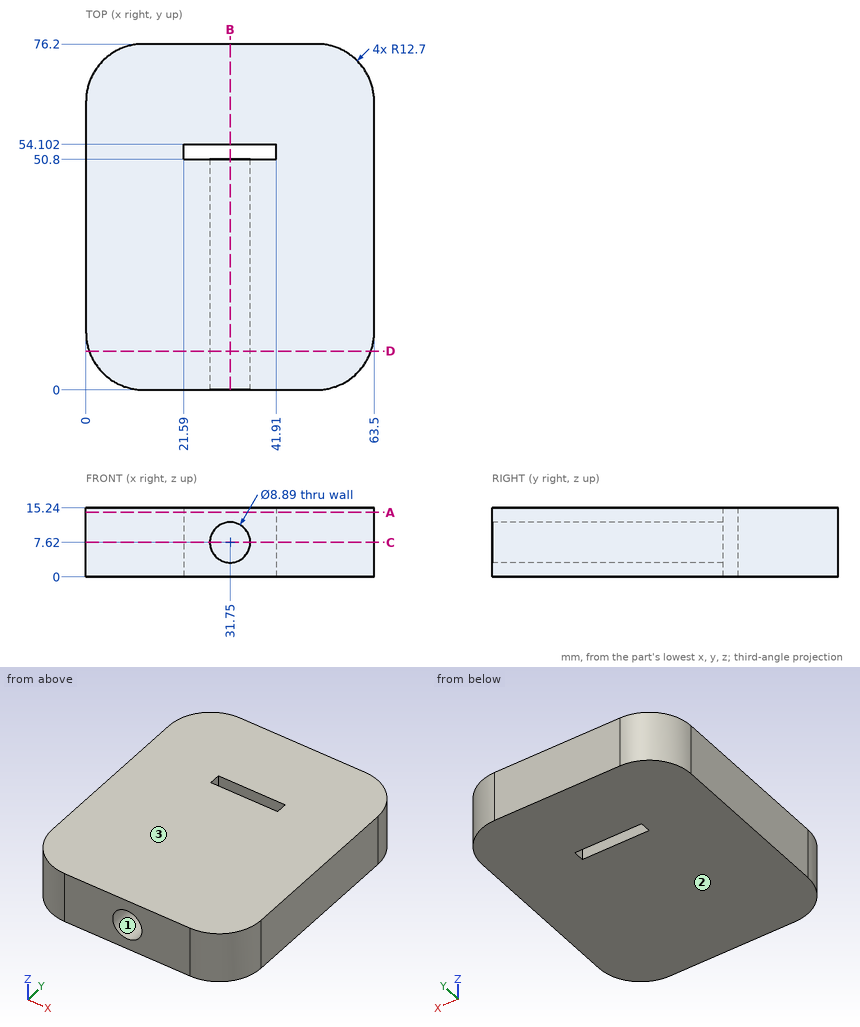
Print and shaded views of the part. All mm, measured from the part's lowest x, y and z. Coordinates: 2 decimals unless noted, no trailing zeros. Loops run counter-clockwise (first coordinate to the right, second up) from the corner with the lowest first, then second, coordinate; pieces in that order, holes last. Notation, with made-up numbers: (5, 23.25) - (60, 23.25) arc R17 ccw to (60, 36.25) - close; hole circle Ø2 at (80.5, -27.5). An arc over 180 degrees is marked (long way). Write item = value, one per line. Start each with the question number.
Item 1: Wall check: L1, parallel to Y at x = 41, z = 6.5; L2, parallel to Z at x = 31.75, y = 37 (3 decimals); L3, parallel to X at y = 30.5, z = 8. Give the ranges that are in metal, low to high. Write a range as from..to.
Item 2: Flat gauge pins, fed straight in: pin 1 Ø3 at (x, z) = (55, 13.5) entering from +Y; pin 2 Ø4 at (x, z) = (6.5, 13.5) entering from -Y; pin 3 Ø1 at (x, z) = (10, 7.5) entering from -Y. Where does each tip first touch, or does it go through?
Item 3: Cut at D-D, the plane y = 8.5. Give the cut face in (x, z) (3 decimals), and give its area (3 significant figures).
Item 4: Cut at C-C, the plane z = 7.62. Give the cut face in (x, y) (3 decimals).
Item 5: Cut at A-A, the plane z = 14.25. Give the cut face in (x, y), and give its area (3 significant figures).
Item 6: Mould opens along Z. For the marked faces 1, 2 and 3 say: released by +Z, released by -Z, zero draft, split by the parting line, or undercut.
Item 7: Cut at B-B, the plane x = 31.75. Give the cut face in (y, z) (3 decimals).
The answers:
q1.L1 = 0..50.8, 54.1..76.2
q1.L2 = 0..3.175, 12.065..15.24
q1.L3 = 0..27.32, 36.18..63.5
q2.pin_1 = 75.91
q2.pin_2 = 0.71
q2.pin_3 = 0.19
q3.outline = (0.715, 0) - (62.785, 0) - (62.785, 15.24) - (0.715, 15.24) - close; hole circle Ø8.89 at (31.75, 7.62)
q3.area = 884 mm2
q4.outline = (0, 12.7) arc R12.7 ccw to (12.7, 0) - (27.305, 0) - (27.305, 50.8) - (21.59, 50.8) - (21.59, 54.102) - (41.91, 54.102) - (41.91, 50.8) - (36.195, 50.8) - (36.195, 0) - (50.8, 0) arc R12.7 ccw to (63.5, 12.7) - (63.5, 63.5) arc R12.7 ccw to (50.8, 76.2) - (12.7, 76.2) arc R12.7 ccw to (0, 63.5) - close
q5.outline = (0, 12.7) arc R12.7 ccw to (12.7, 0) - (50.8, 0) arc R12.7 ccw to (63.5, 12.7) - (63.5, 63.5) arc R12.7 ccw to (50.8, 76.2) - (12.7, 76.2) arc R12.7 ccw to (0, 63.5) - close; hole (21.59, 50.8) - (41.91, 50.8) - (41.91, 54.1) - (21.59, 54.1) - close
q5.area = 4,630 mm2
q6.face_1 = undercut
q6.face_2 = released by -Z
q6.face_3 = released by +Z
q7.outline = (0, 0) - (50.8, 0) - (50.8, 3.175) - (0, 3.175) - close; (0, 12.065) - (50.8, 12.065) - (50.8, 15.24) - (0, 15.24) - close; (54.102, 0) - (76.2, 0) - (76.2, 15.24) - (54.102, 15.24) - close
